from build123d import *

# Parameters (mm, degrees)
SKETCH_1_R          = 4
EXTRUDE_1_DEPTH     = 4
SKETCH_2_R          = 2.5
EXTRUDE_2_DEPTH     = 34
CUT_EXTRUDE_1_DEPTH = 2
CHAMFER_1_SIZE      = 0.2
CHAMFER_2_SIZE      = 0.3


with BuildPart() as part:
    # 草图1 → 凸台-拉伸1 (new body)
    with BuildSketch(Plane(origin=(0, 0, 0), x_dir=(1, 0, 0), z_dir=(0, 1, 0))):
        Circle(SKETCH_1_R)
    extrude(amount=EXTRUDE_1_DEPTH)

    # 草图2 → 凸台-拉伸2 (add)
    with BuildSketch(Plane.XZ):
        Circle(SKETCH_2_R)
    extrude(amount=EXTRUDE_2_DEPTH)

    # 草图11 → 切除-拉伸1 (cut)
    with BuildSketch(Plane(origin=(0, 4, 0), x_dir=(1, 0, 0), z_dir=(0, 1, 0))):
        Polygon((1.154954177, 1.999853541), (-1.154446882, 2.000146427), (-2.309401058, 0.000292887), (-1.154954177, -1.999853541), (1.154446882, -2.000146427), (2.309401058, -0.000292887), align=None)
    extrude(amount=-CUT_EXTRUDE_1_DEPTH, mode=Mode.SUBTRACT)

    # 倒角1
    chamfer_1_edges = [part.edges().sort_by_distance(p)[0] for p in [
        (1.732177617, 4, -0.999780327),
        (0.000253647, 4, -1.999999984),
        (-1.73192397, 4, -1.000219657),
        (-1.732177617, 4, 0.999780327),
        (-0.000253647, 4, 1.999999984),
        (1.73192397, 4, 1.000219657),
        (-4, 4, 0),
    ]]
    chamfer(chamfer_1_edges, length=CHAMFER_1_SIZE)

    # 倒角2
    chamfer_2_edges = [part.edges().sort_by_distance(p)[0] for p in [
        (-2.5, -34, 0),
    ]]
    chamfer(chamfer_2_edges, length=CHAMFER_2_SIZE)


solid = part.part
Input: part model. Units: mm. Frame: model coordinates. A direction names the side the tool comes from. Coordinates: 2 decimals unless noted, no trailing zeros. Order: outer loops, then holes, each group sorted by start corner. A loop starts at its lowest first (then second) coordinate and runs counter-clockwise, first axis right, second up. Notation, with made-up numbers: M -1.5,74 L 7.5,74 A19 cw 7.5,93 Z; hole C -38.75,58 d1. An arc over 180 degrees is marked long. One line per question, with ' | ' between items.
Item 1: Pin query (flat end, axial travel): pin 1 (1.5 mm diameter, centred on y = -21.5, z = 2.5, fed in from +X); pin 2 (1 mm diameter, centred on x = 1.5, y = -17, fed in from -Z). Return the tip coordinate at first contact, or that it passes through.
Geometry results:
pin 1: stops at x = 1.79 | pin 2: stops at z = -2.29
Item 2: Reachability of faces 1 (the flat face through (-1.724, 2.913, -1.014)), 2 (the flat face through (2, 0, -2)), 3 (the flat face through (2, 4, 2)) from +Z, -Z, +X, -X, +Y, -Y: full face, straight path, thin tool, end or side. Return the list, or none.
Geometry results:
face 1: +Y | face 2: -Y | face 3: +Z, -Z, +X, -X, +Y
Item 3: Section B-B (y = -8). Output: boundary loops of the cut face in (x, z).
Geometry results:
outline: C 0,0 d5
Item 4: Ray query, line 1 along Y through (x, z) = (3, -1); line 2 along Y through (x, z) = (1.25, 0.5); line 3 along Z through (x, y) = (-1.75, 1). Return the intervals inside material, ascending.
Geometry results:
line 1: y = 0 to 4 | line 2: y = -34 to 2 | line 3: z = -3.6 to 3.6
Item 5: Draft query along Z for faces 4 (the flat face through (1.74, 2.91, -0.99)), 5 (the flat face through (0, -34, 0)), 6 (the cylindrical face through (-0.867, 1.873, 3.905)). Return one class per face: released by +Z, released by -Z, zero draft, split by the parting line, or undercut.
Geometry results:
face 4: undercut | face 5: zero draft | face 6: split by the parting line
Item 6: Section A-A (x = 0). Output: boundary loops of the cut face in (y, z), then the cut area to 3 significant figures.
Geometry results:
outline: M -34,-2.2 L -33.7,-2.5 L 0,-2.5 L 0,-4 L 3.8,-4 L 4,-3.8 L 4,-2.2 L 3.8,-2 L 2,-2 L 2,2 L 3.8,2 L 4,2.2 L 4,3.8 L 3.8,4 L 0,4 L 0,2.5 L -33.7,2.5 L -34,2.2 Z | area: 194 mm^2
